Read the model definition and answer for the solid it produces. Units are mm, in the model's axes. Give positions to 0.01 mm unless a question says otherwise; leave off trailing zeros. Use one line per item in the form item = value.
```python
from build123d import *

# Parameters (mm, degrees)
F0_W      = 400
F0_H      = 350
F1_DEPTH  = 19
F3_DEPTH  = 19.001
F5_DEPTH  = 19.0010001
F8_DEPTH  = 19.0010001
F9_R      = 22.041602622
F10_DEPTH = 19.0010001


with BuildPart() as f1:
    # F0 (on Top) → F1 (new body)
    with BuildSketch(Plane.XY):
        Rectangle(F0_W, F0_H)
    extrude(amount=F1_DEPTH)

    # F2 (on face) → F3 (cut, through all)
    with BuildSketch(Plane.XY.offset(19)):
        with BuildLine():
            Line((-200, 175), (-200, 0))
            add(Edge.make_bspline(
                [(-200, 0), (-197.9354059876, 47.0718279126), (-194.3381993041, 129.0865450701), (-116.4199550867, 173.9492192316), (-112.5868335366, 175)],
                knots=[0, 0, 0, 0, 0.5533709859, 0.9641555662, 0.9641555662, 0.9641555662, 0.9641555662], degree=3))
            Line((-112.5868335366, 175), (-200, 175))
        make_face()
    extrude(amount=-F3_DEPTH, mode=Mode.SUBTRACT)

    # F4 (on face) → F5 (cut, through all)
    with BuildSketch(Plane.XY.offset(19)):
        with BuildLine():
            add(Edge.make_bspline(
                [(200, 0), (186.7244970993, 49.4813033152), (163.5787269472, 135.7516978857), (111.7638804337, 163.2665740198), (89.6679908037, 175)],
                knots=[0, 0, 0, 0, 0.5735606469, 1, 1, 1, 1], degree=3))
            Line((200, 0), (200, 175))
            Line((200, 175), (89.6679908037, 175))
        make_face()
    extrude(amount=-F5_DEPTH, mode=Mode.SUBTRACT)

    # F6 (on face) + F7 (on face) → F8 (cut, through all)
    with BuildSketch(Plane.XY.offset(19)):
        with BuildLine():
            Line((-200, -175), (0, -175))
            add(Edge.make_bspline(
                [(0, -175), (-47.4363116832, -162.5537951207), (-135.1863297266, -139.5301943393), (-179.5970382425, -83.2807067772), (-200, -57.4388280511)],
                knots=[0, 0, 0, 0, 0.5405846374, 1, 1, 1, 1], degree=3))
            Line((-200, -57.4388280511), (-200, -175))
        make_face()
    with BuildSketch(Plane.XY.offset(19)):
        with BuildLine():
            add(Edge.make_bspline(
                [(0.6422742583, -175), (55.1586444169, -162.6567958418), (148.7558794279, -141.3724859979), (184.9953796241, -92.3328411017), (200, -71.7412712825)],
                knots=[0.0022640226, 0.0022640226, 0.0022640226, 0.0022640226, 0.5787782178, 0.9934410048, 0.9934410048, 0.9934410048, 0.9934410048], degree=3))
            Line((0.6422742583, -175), (200, -175))
            Line((200, -175), (200, -71.7412712825))
        make_face()
    extrude(amount=-F8_DEPTH, mode=Mode.SUBTRACT)

    # F9 (on face) → F10 (cut, through all)
    with BuildSketch(Plane.XY.offset(19)):
        with Locations((-8.6059067398, 143.5507237911)):
            Circle(F9_R)
    extrude(amount=-F10_DEPTH, mode=Mode.SUBTRACT)


solid = f1.part
```
Item 1: Given pin 1 Ø10 at (y, z) = (110, 8.5) entering from -X; pin 2 Ø1 at (x, z) = (85.5, 3.5) entering from -Y; pin 3 Ø2 at (y, z) = (6, 8) entering from +X, each flat-ended and moving along its own axis, determine where each tip first touches the part or whether it passes through.
Checks:
pin_1 = -183.27
pin_2 = -153.76
pin_3 = 198.66
Item 2: Straight lines are drawn through the part: L1, parallel to Y at x = -27.5, z = 13.75; L2, parallel to Y at x = -178.5, z = 4.5; L3, parallel to Y at x = -71.5, z = 3.5. For each, find the intervals that lie inside material, in ascending order. Write a range as from..to.
Checks:
L1 = -167.69..132.2, 154.9..175
L2 = -83.91..114.78
L3 = -154.46..175
Item 3: Determine the mould class of faces 1 (the cylindrical face through (-11.5, 165.4, 9.6)), 2 (the flat face through (-13, 175, 9)), 3 (the flat face through (200, -36, 9)) for opening direction X: +X half, -X half, draft (parallel to the pull), parting line (faces both ways), or undercut.
Checks:
face_1 = undercut
face_2 = draft
face_3 = +X half
